CAD build for the part. Positions are in the model's coordinates, mm. A direction names the side the tool comes from. Round coordinates to 2 decimals unless told otherwise and drop trailing zeros. Order: outer loops, then holes, each group sorted by start corner. A loop starts at its lowest first (then second) coordinate and runs counter-clockwise, first axis right, second up. Notation, with made-up numbers: (52.25, 80) -> (101.25, 80) arc R22 cw to (101.25, 117) -> close; hole circle Ø7 at (-1, 24.25). An arc over 180 degrees is marked (long way). Answer as CSV lines item,"result". Start each with the question number.
from build123d import *

# Parameters (mm, degrees)
F0_W      = 16
F0_H      = 25
F0_R      = 5
F1_DEPTH  = 2
F2_W      = 3
F2_H      = 25
F3_DEPTH  = 3
F4_W      = 3
F4_H      = 25
F5_DEPTH  = 65
F6_W      = 3
F6_H      = 25
F7_DEPTH  = 70
F10_DEPTH = 67
F11_W     = 3
F11_H     = 25
F12_DEPTH = 80
F13_R     = 2.5
F14_DEPTH = 3
F16_DEPTH = 16.001
F17_W     = 1
F17_H     = 67
F18_DEPTH = 9
F19_W     = 1
F19_H     = 73
F20_DEPTH = 25.001


with BuildPart() as f1:
    # F0 (on Front) → F1 (new body)
    with BuildSketch(Plane.XZ):
        with Locations((-20.477814, -3.461555)):
            Rectangle(F0_W, F0_H)
        with Locations((-20.477814, 3.038445)):
            Circle(F0_R, mode=Mode.SUBTRACT)
    extrude(amount=F1_DEPTH)

    # F2 (on face) → F3 (join)
    with BuildSketch(Plane.XZ.offset(2)):
        with Locations((-13.977814, -3.461555)):
            Rectangle(F2_W, F2_H)
    extrude(amount=F3_DEPTH)

    # F4 (on face) → F5 (join)
    with BuildSketch(Plane.YZ.offset(-12.477814)):
        with Locations((-3.5, -3.461555)):
            Rectangle(F4_W, F4_H)
    extrude(amount=F5_DEPTH)

    # F6 (on face) → F7 (join)
    with BuildSketch(Plane(origin=(0, -2, 0), x_dir=(-1, 0, 0), z_dir=(0, 1, 0))):
        with Locations((-51.022186, -3.461555)):
            Rectangle(F6_W, F6_H)
    extrude(amount=F7_DEPTH)

    # F9 (on face) → F10 (join)
    with BuildSketch(Plane(origin=(0, -2, 0), x_dir=(-1, 0, 0), z_dir=(0, 1, 0))):
        Polygon((-49.522186, 0.038445), (-49.522186, -15.961555), (-44.522186, -15.961555), (-24.522186, -4.961555), (-24.522186, 0.038445), align=None)
    extrude(amount=F10_DEPTH)

    # F11 (on face) → F12 (join)
    with BuildSketch(Plane(origin=(49.522186, 0, 0), x_dir=(0, -1, 0), z_dir=(-1, 0, 0))):
        with Locations((-66.5, -3.461555)):
            Rectangle(F11_W, F11_H)
    extrude(amount=F12_DEPTH)

    # F13 (on face) → F14 (cut)
    with BuildSketch(Plane(origin=(0, 68, 0), x_dir=(-1, 0, 0), z_dir=(0, 1, 0))):
        with Locations((20.477814, 3.038445)):
            Circle(F13_R)
    extrude(amount=-F14_DEPTH, mode=Mode.SUBTRACT)

    # F15 (on face) → F16 (cut, through all)
    with BuildSketch(Plane.XY.offset(0.038445)):
        Polygon((31.522186, 62), (24.522186, 62), (24.522186, 8), align=None)
    extrude(amount=-F16_DEPTH, mode=Mode.SUBTRACT)

    # F17 (on face) → F18 (join, through all)
    with BuildSketch(Plane.XY.offset(0.038445)):
        with Locations((49.022186, 31.5)):
            Rectangle(F17_W, F17_H)
    extrude(amount=F18_DEPTH)

    # F19 (on face) → F20 (cut, through all)
    with BuildSketch(Plane.XY.offset(9.038445)):
        with Locations((52.022186, 31.5)):
            Rectangle(F19_W, F19_H)
    extrude(amount=-F20_DEPTH, mode=Mode.SUBTRACT)


solid = f1.part
Item 1: Band-saw the part on D-D, the plane x = -22. Give the cut face in (y, z), and give its area (3 significant figures).
Item 2: Mould opens along X. For faces 6 (the flat face through (-12.478, -1, -4)), 7 (the flat face through (-21, 0, -6)), 8 (the flat face through (24.522, 63, -2)) say: released by +X, released by -X, zero draft, split by the parting line, or undercut.
Item 3: Band-saw the part on A-A, the plane x = -11.5. Give the cut face in (y, z), and give its area (3 significant figures).
Item 4: Band-saw the part on B-B, the plane y = 3. Give the cut face in (x, z), and give its area (3 significant figures).
Item 5: Pin check, flat tips, straight feed: pin 1 (12 mm diameter, centred on x = 33.5, y = 39, fed in from +Z); pin 2 (12 mm diameter, centred on y = 15, z = -8, fed in from -X); pin 3 (6 mm diameter, centred on x = -20.48, z = 3.04, fed in from -Y). Stop position of each tip, or through.
Item 6: Probe line 1 (Y direction, x = -15, z = 7.75); line 2 (Y direction, x = 13.5, z = -14); line 3 (X direction, y = 26, z = 3.5). List the from-to ranges inside material, lowest first.
Item 7: Band-saw the part on C-C, the plane z = 4.5. Give the cut face in (x, y).
Item 8: Tool access for faces 1 (the flat face through (24.522, 3, -2)), 2 (the flat face through (27.973, 34.622, -3.341)), 3 (the cylindrical face through (-22.862, 66.521, 3.789)), 4 (the flat face through (-15.478, -3, -4)), 5 (the flat face through (47, 34, -15.962)): list every direction of +Z, -Z, +X, -X, +Y, -Y with a clear straight run to the whole face (end or side of a thin tool).
Values:
1,outline,"(-2, -15.96) -> (0, -15.96) -> (0, -1.72) -> (-2, -1.72) -> close; (-2, 7.8) -> (0, 7.8) -> (0, 9.04) -> (-2, 9.04) -> close; (65, -15.96) -> (68, -15.96) -> (68, 1.06) -> (65, 1.06) -> close; (65, 5.02) -> (68, 5.02) -> (68, 9.04) -> (65, 9.04) -> close"
1,area,"94.1 mm²"
2,face 6,"undercut"
2,face 7,"zero draft"
2,face 8,"released by -X"
3,outline,"(-5, -15.96) -> (-2, -15.96) -> (-2, 9.04) -> (-5, 9.04) -> close; (65, -15.96) -> (68, -15.96) -> (68, 9.04) -> (65, 9.04) -> close"
3,area,"150 mm²"
4,outline,"(24.52, -4.96) -> (44.52, -15.96) -> (51.52, -15.96) -> (51.52, 9.04) -> (48.52, 9.04) -> (48.52, 0.04) -> (24.52, 0.04) -> close"
4,area,"349 mm²"
5,pin 1,"z = 0.04"
5,pin 2,"x = 24.75"
5,pin 3,"y = 65"
6,line 1,"-5 to 0, 65 to 68"
6,line 2,"-5 to -2, 65 to 68"
6,line 3,"48.52 to 51.52"
7,outline,"(-30.48, 65) -> (-22.51, 65) -> (-22.51, 68) -> (-30.48, 68) -> close; (-28.48, -2) -> (-25.26, -2) -> (-25.26, 0) -> (-28.48, 0) -> close; (-18.45, 65) -> (48.52, 65) -> (48.52, -2) -> (-12.48, -2) -> (-12.48, 0) -> (-15.7, 0) -> (-15.7, -2) -> (-15.48, -2) -> (-15.48, -5) -> (51.52, -5) -> (51.52, 68) -> (-18.45, 68) -> close"
8,face 1,"+Z, -Z"
8,face 2,"+Z, -Z, -X"
8,face 3,"+Y, -Y"
8,face 4,"+Z, -Z, -X, -Y"
8,face 5,"-Z, +X, -X, +Y, -Y"
